Verification items for the finished model (mm, model axes). Face numbers are marked on the shaded views. A direction names the side the tool comes from. Give positions to 0.01 mm unless a question says otherwise; leave off trailing zeros. Loops run counter-clockwise (first coordinate to the right, second up) from the corner with the lowest first, then second, coordinate; pieces in that order, holes last. Notation, with made-up numbers: (4, 8.25) - (59, 8.25) arc R20 cw to (59, 41.25) - close; hole circle Ø3 at (73, 68). An arc over 180 degrees is marked (long way). Answer in a Markdown table with one row per item.
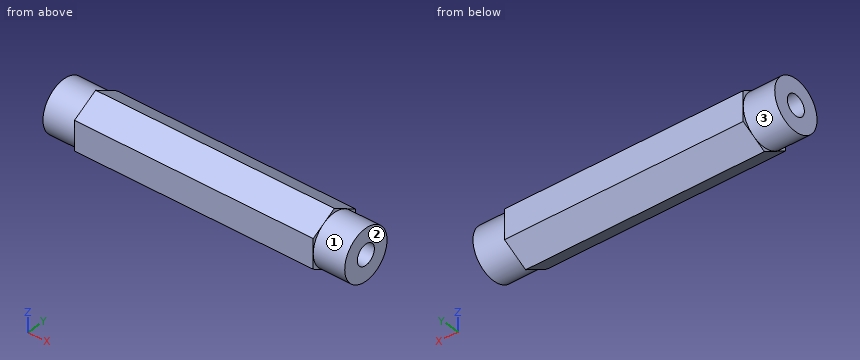
Autodesk Inventor part; units mm, degrees
ref_plane "YZ Plane" through (0, 0, 0) normal (1, 0, 0) x (0, 1, 0)
ref_plane "XZ Plane" through (0, 0, 0) normal (0, 1, 0) x (-1, 0, 0)
ref_plane "XY Plane" through (0, 0, 0) normal (0, 0, 1) x (1, 0, 0)
sketch "Sketch1" plane through (0, 0, 0) normal (1, 0, 0) x (0, 1, 0)
  line L0 (0, -7.3323) -> (-6.35, -3.6662)
  line L1 (-6.35, -3.6662) -> (-6.35, 3.6662)
  line L2 (-6.35, 3.6662) -> (0, 7.3323)
  line L3 (0, 7.3323) -> (6.35, 3.6662)
  line L4 (6.35, 3.6662) -> (6.35, -3.6662)
  line L5 (6.35, -3.6662) -> (0, -7.3323)
  point P0 (0, 0)
  point P1 (0, 0)
  dimension "d0" = 12.7
extrude "Extrusion1" add sketch "Sketch1" along normal mid plane 60.2996
sketch "Sketch2" plane through (-30.1498, 0, 0) normal (-1, 0, 0) x (0, 0, 1)
  circle A0 centre (0, 0) radius 6.35
  dimension "d3" = 12.7
extrude "Extrusion2" add sketch "Sketch2" along normal blind 7.9502
sketch "Sketch3" plane through (30.1498, 0, 0) normal (1, 0, 0) x (0, 0, -1)
  circle A0 centre (0, 0) radius 6.35
  line L0 (3.6662, 6.35) -> (-3.6662, 6.35)
  line L1 (-3.6662, 6.35) -> (-7.3323, 0)
  line L2 (-7.3323, 0) -> (-3.6662, -6.35)
  line L3 (-3.6662, -6.35) -> (3.6662, -6.35)
  line L4 (3.6662, -6.35) -> (7.3323, 0)
  line L5 (7.3323, 0) -> (3.6662, 6.35)
  dimension "d6" = 12.7
extrude "Extrusion3" add sketch "Sketch3" along normal blind 7.9502 contours A0
sketch "Sketch4" plane through (38.1, 0, 0) normal (1, 0, 0) x (0, 0, -1)
  point P0 (0, 0)
  point P1 (0, 0)
hole "Hole1" at (38.1, 0, 0) direction (-1, 0, 0) diameter 5.1054 end through all
properties part number "EL2-GB-003" material "Aluminum 6061"
Q1. Sectioned sample at B-B (z = 1.25). Record the cut outline in (x, y).
Completed:
| item | result |
|---|---|
| outline | (-38.1, -6.23) - (-30.15, -6.23) - (-30.15, -6.35) - (30.15, -6.35) - (30.15, -6.23) - (38.1, -6.23) - (38.1, -2.23) - (-38.1, -2.23) - close; (-38.1, 2.23) - (38.1, 2.23) - (38.1, 6.23) - (30.15, 6.23) - (30.15, 6.35) - (-30.15, 6.35) - (-30.15, 6.23) - (-38.1, 6.23) - close |
Q2. Thickness scan on line 1 (Y direction, x = -7, z = 0); line 2 (Z direction, x = -20, y = 0); line 3 (Z direction, x = 30.5, y = -2.25). Record the ranges inside material, lowest first.
Completed:
| item | result |
|---|---|
| line 1 | -6.35 to -2.55, 2.55 to 6.35 |
| line 2 | -7.33 to -2.55, 2.55 to 7.33 |
| line 3 | -5.94 to -1.21, 1.21 to 5.94 |
Q3. Sectioned sample at A-A (x = 4). Record the cut outline in (y, z), and give its area (3 significant figures).
Completed:
| item | result |
|---|---|
| outline | (-6.35, -3.67) - (0, -7.33) - (6.35, -3.67) - (6.35, 3.67) - (0, 7.33) - (-6.35, 3.67) - close; hole circle Ø5.11 at (0, 0) |
| area | 119 mm^2 |
Q4. Go/stop test with flat-tipped pins: P1, Ø3, axis at x = 0.5, y = 2, coming from the -Z side; P2, Ø5, axis at x = -13, y = 4, coming from the +Z side; P3, Ø1.5, axis at x = 30, y = 1.5, coming from the +Z side. Record where each tip stops, or that it passes through.
Completed:
| item | result |
|---|---|
| P1 | z = -7.04 |
| P2 | z = 6.47 |
| P3 | z = 6.9 |
Q5. Sectioned sample at D-D (y = 4). Record the cut outline in (x, z).
Completed:
| item | result |
|---|---|
| outline | (-38.1, -4.93) - (-30.15, -4.93) - (-30.15, -5.02) - (30.15, -5.02) - (30.15, -4.93) - (38.1, -4.93) - (38.1, 4.93) - (30.15, 4.93) - (30.15, 5.02) - (-30.15, 5.02) - (-30.15, 4.93) - (-38.1, 4.93) - close |
Q6. Tool access check on the marked faces 1, 2 and 3. Record the directions out of +Z, -Z, +X, -X, +Y, -Y that give a thin tool (end or side, any length) a straight path to the whole face; none if there is none.
Completed:
| item | result |
|---|---|
| face 1 | +X |
| face 2 | +Z, -Z, +X, +Y, -Y |
| face 3 | -X |
Q7. Sectioned sample at C-C (y = 0.75). Record the cut outline in (x, z), and give its area (3 significant figures).
Completed:
| item | result |
|---|---|
| outline | (-38.1, -6.31) - (-30.15, -6.31) - (-30.15, -6.9) - (30.15, -6.9) - (30.15, -6.31) - (38.1, -6.31) - (38.1, -2.44) - (-38.1, -2.44) - close; (-38.1, 2.44) - (38.1, 2.44) - (38.1, 6.31) - (30.15, 6.31) - (30.15, 6.9) - (-30.15, 6.9) - (-30.15, 6.31) - (-38.1, 6.31) - close |
| area | 661 mm^2 |
